The model under review builds one solid part; all positions refer to its coordinate system, in mm. A direction names the side the tool comes from. Give positions to 0.01 mm unless a question says otherwise; leave off trailing zeros. Write each loop counter-clockwise with the first axis right and the second up, starting at its lowest first coordinate (ties: lowest second). Pieces come first, ordered by that corner, then holes. Notation, with made-up numbers: (64.25, 40) - (78.25, 40) arc R35 ccw to (78.25, 79) - close; hole circle Ø3 at (-32.75, -22). An arc over 180 degrees is marked (long way). Write item = value, one per line.
```python
from build123d import *

# Parameters (mm, degrees)
BOSS_EXTRUDE1_DEPTH    = 3.175
CUT_EXTRUDE1_DEPTH     = 66.066884919
CUT_EXTRUDE2_DEPTH     = 65.107450137
BOSS_EXTRUDE2_DEPTH    = 6.35
M3_5_CLEARANCE_HOLE1_D = 3.81
FILLET1_R              = 3.175
FILLET2_R              = 6.35


with BuildPart() as part:
    # Sketch1 → Boss-Extrude1 (new body)
    with BuildSketch(Plane.XY.offset(3.175)):
        Polygon((54.97356176, 15.279413628), (-2.152444785, 34.663040771), (-18.475499222, -13.443070004), (38.650507323, -32.826697147), align=None)
    extrude(amount=-BOSS_EXTRUDE1_DEPTH)

    # Sketch2 → Cut-Extrude1 (cut, through all)
    with BuildSketch(Plane(origin=(0, 0, 0), x_dir=(-1, 0, 0), z_dir=(0, 0, -1))):
        Polygon((2.152444785, 34.663040771), (-6.867450985, 31.602468064), (-0.746305571, 13.562676524), (8.273590199, 16.62324923), align=None)
    extrude(amount=-CUT_EXTRUDE1_DEPTH, mode=Mode.SUBTRACT)

    # Sketch3 → Cut-Extrude2 (cut, through all)
    with BuildSketch(Plane(origin=(0, 0, 0), x_dir=(-1, 0, 0), z_dir=(0, 0, -1))):
        Polygon((18.475499222, -13.443070004), (12.354353808, 4.596721537), (3.334458038, 1.53614883), (9.455603451, -16.503642711), align=None)
    extrude(amount=-CUT_EXTRUDE2_DEPTH, mode=Mode.SUBTRACT)

    # Sketch4 → Boss-Extrude2 (add)
    with BuildSketch(Plane.XY.offset(3.175)):
        Polygon((46.919916108, 11.306531586), (34.677625281, -24.773051496), (-1.4019578, -12.530760668), (10.840333027, 23.548822413), align=None)
    extrude(amount=BOSS_EXTRUDE2_DEPTH)

    # M3.5 Clearance Hole1 (through all)
    with Locations(Plane.XY.offset(3.175)):
        with Locations((-6.826278972, 9.426563937)):
            Hole(M3_5_CLEARANCE_HOLE1_D / 2)

    # Fillet1
    fillet1_edges = [part.edges().sort_by_distance(p)[0] for p in [
        (-8.273590199, 16.62324923, 1.5875),
        (0.746305571, 13.562676524, 1.5875),
        (6.867450985, 31.602468064, 1.5875),
        (-9.455603451, -16.503642711, 1.5875),
        (-3.334458038, 1.53614883, 1.5875),
        (-12.354353808, 4.596721537, 1.5875),
        (38.650507323, -32.826697147, 1.5875),
        (54.97356176, 15.279413628, 1.5875),
    ]]
    fillet(fillet1_edges, radius=FILLET1_R)

    # Fillet2
    fillet2_edges = [part.edges().sort_by_distance(p)[0] for p in [
        (46.919916108, 11.306531586, 6.35),
        (10.840333027, 23.548822413, 6.35),
        (-1.4019578, -12.530760668, 6.35),
        (34.677625281, -24.773051496, 6.35),
    ]]
    fillet(fillet2_edges, radius=FILLET2_R)


solid = part.part
```
1. Take a section at B-B on x = 44. Give the boundary of the cut face in (y, z) (3 decimals), and give its area (3 significant figures).
Findings below:
outline = (-17.061, 0) - (19.003, 0) - (19.003, 3.175) - (11.071, 3.175) - (11.071, 9.525) - (2.701, 9.525) - (2.701, 3.175) - (-17.061, 3.175) - close
area = 168 mm²
2. Machinability: for faces 1 (the cylindrical face through (12.07, 21.22, 6.39)), 2 (the flat face through (16.81, -18.71, 6.31)), 3 (the flat face through (40.856, -6.565, 6.306)), 4 (the flat face through (28.712, 17.485, 6.306)), which of the approach directions +Z, -Z, +X, -X, +Y, -Y give a long, thin tool a straight path to every point of the face, cutting with its end or side? Answer none if there is none.
Findings below:
face_1 = +Z, +Y
face_2 = +Z, -X, -Y
face_3 = +Z, +X, -Y
face_4 = +Z, +X, +Y
3. For line 1 (Z direction, x = 18, y = -19.5) (3 decimals); line 2 (Y direction, x = 22.5, z = 8); line 3 (X direction, y = -3, z = 6.5), list the stretches that pass through material, from the lowest coordinate up. Write a range as from..to.
Findings below:
line_1 = 0..3.175
line_2 = -20.64..19.59
line_3 = 1.83..42.07
4. Draft analysis for pull direction X (two halves, no side actions). For faces 5 (the flat face through (46.7, -9.1, 1.6)), 6 (the cylindrical face through (-5.42, 10.71, 1.57)), 7 (the cylindrical face through (0.2, 14.76, 1.61)), 8 (the flat face through (-7.865, 3.074, 1.565)), state which applies: +X half, -X half, draft (parallel to the pull), parting line (faces both ways), or undercut.
Findings below:
face_5 = +X half
face_6 = undercut
face_7 = undercut
face_8 = -X half
5. Take a section at A-A on z = 8.75. Give the boundary of the cut face in (x, y).
Findings below:
outline = (0.64, -6.52) arc R6.35 ccw to (4.61, -14.57) - (28.66, -22.73) arc R6.35 ccw to (36.72, -18.76) - (44.88, 5.29) arc R6.35 ccw to (40.91, 13.35) - (16.85, 21.51) arc R6.35 ccw to (8.8, 17.54) - close
6. Insertion check: P1, Ø4, axis at y = -5, z = 6.5, coming from the +X side; P2, Ø3.5, axis at x = -6.83, y = 9.43, coming from the +Z side; P3, Ø4, axis at x = 35.5, z = 6, coming from the +Y side; P4, Ø1, axis at y = 1.5, z = 2, coming from the -X side. Each pin has a flat end and moves straight along its axis. Give the tip position at first contact, or say it passes through.
Findings below:
P1 = 42.07
P2 = through
P3 = 15.86
P4 = -5.34
